For this review, take the finished solid that the model builds, in its own axes (mm). Face numbers are marked on the shaded views. A direction names the side the tool comes from. Round coordinates to 2 decimals unless told otherwise and drop trailing zeros. Order: outer loops, then holes, each group sorted by start corner. A loop starts at its lowest first (then second) coordinate and runs counter-clockwise, first axis right, second up. Notation, with made-up numbers: M 8.5,-12 L 43.5,-12 A10 cw 43.5,-2 Z; hole C -35.5,3.5 d10. An arc over 180 degrees is marked long. Put each result on its own line as item: value.
from build123d import *

# Parameters (mm, degrees)
F1_DEPTH       = 101.6
F3_D           = 9.525
F3_DEPTH       = 15.875
F3_CBORE_D     = 9.525
F3_CBORE_DEPTH = 9.525
F3_TIP         = 2.8615986981
F5_D           = 9.525
F5_CBORE_D     = 12.7
F5_CBORE_DEPTH = 12.7
F6_W           = 38.1
F6_H           = 38.1
F7_DEPTH       = 57.913
F8_R           = 9.525
F9_DEPTH       = 31.751


with BuildPart() as f1:
    # F0 (on Right) → F1 (new body)
    with BuildSketch(Plane.YZ):
        with BuildLine():
            Line((-18.288, 0), (-32.512, 0))
            Line((-32.512, 0), (-32.512, -31.75))
            Line((-32.512, -31.75), (-26.162, -31.75))
            ThreePointArc((-26.162, -31.75), (-24.3021280605, -27.2598719395), (-19.812, -25.4))
            Line((-19.812, -25.4), (19.812, -25.4))
            ThreePointArc((19.812, -25.4), (24.3021280605, -27.2598719395), (26.162, -31.75))
            Line((26.162, -31.75), (32.512, -31.75))
            Line((32.512, -31.75), (32.512, 0))
            Line((32.512, 0), (18.288, 0))
            Line((18.288, 0), (18.288, 6.35))
            Line((18.288, 6.35), (25.4, 6.35))
            Line((25.4, 6.35), (25.4, 38.1))
            Line((25.4, 38.1), (19.05, 38.1))
            Line((19.05, 38.1), (3.302, 22.352))
            Line((3.302, 22.352), (3.302, 16.002))
            Line((3.302, 16.002), (-3.302, 16.002))
            Line((-3.302, 16.002), (-3.302, 22.352))
            Line((-3.302, 22.352), (-19.05, 38.1))
            Line((-19.05, 38.1), (-25.4, 38.1))
            Line((-25.4, 38.1), (-25.4, 6.35))
            Line((-25.4, 6.35), (-18.288, 6.35))
            Line((-18.288, 6.35), (-18.288, 0))
        make_face()
    extrude(amount=-F1_DEPTH)

    # F3
    with Locations(Plane.YZ):
        with Locations((0, -9.525)):
            CounterBoreHole(F3_D / 2, F3_CBORE_D / 2, F3_CBORE_DEPTH, depth=F3_DEPTH)
            with Locations((0, 0, -(F3_DEPTH + F3_TIP / 2))):  # 118° drill point
                Cone(0, F3_D / 2, F3_TIP, mode=Mode.SUBTRACT)

    # F5 (through all)
    with Locations(Plane.XZ.offset(32.512)):
        with Locations((-50.8, -15.875)):
            CounterBoreHole(F5_D / 2, F5_CBORE_D / 2, F5_CBORE_DEPTH)

    # F6 (on face) → F7 (cut, through all)
    with BuildSketch(Plane.XZ.offset(25.4)):
        with Locations((-50.8, 19.05)):
            Rectangle(F6_W, F6_H)
    extrude(amount=-F7_DEPTH, mode=Mode.SUBTRACT)

    # F8 (on face) → F9 (cut, through all)
    with BuildSketch(Plane.XY):
        with Locations((-50.8, 0)):
            Circle(F8_R)
    extrude(amount=-F9_DEPTH, mode=Mode.SUBTRACT)


solid = f1.part
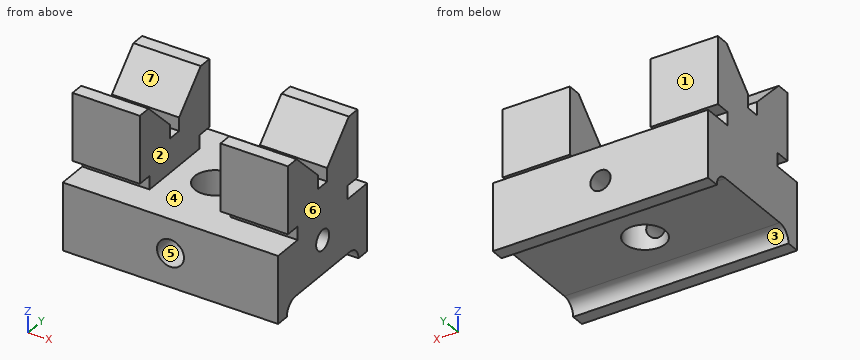
(1) Add section A-A on z = 4. Give the boundary of the cut face in (x, y).
A:
outline: M -101.6,-18.29 L -69.85,-18.29 L -69.85,18.29 L -101.6,18.29 Z; M -31.75,-18.29 L 0,-18.29 L 0,18.29 L -31.75,18.29 Z
(2) Add section B-B on z = 33. Give the boundary of the cut face in (x, y).
A:
outline: M -101.6,-25.4 L -69.85,-25.4 L -69.85,-13.95 L -101.6,-13.95 Z; M -101.6,13.95 L -69.85,13.95 L -69.85,25.4 L -101.6,25.4 Z; M -31.75,-25.4 L 0,-25.4 L 0,-13.95 L -31.75,-13.95 Z; M -31.75,13.95 L 0,13.95 L 0,25.4 L -31.75,25.4 Z
(3) To check wall thickness, follow L1, parallel to Z at x = -10.75, y = 0; L2, parallel to X at y = -6, z = 5; L3, parallel to Z at x = -92, y = 1. State the ranges of each line that lie inside material, in increasing order.
A:
L1: z = -25.4 to -14.29, -4.76 to 16
L2: x = -101.6 to -69.85, -31.75 to 0
L3: z = -25.4 to 16
(4) Add section D-D on y = -7. Give the boundary of the cut face in (x, z), then the cut area to 3 significant figures.
A:
outline: M -101.6,-25.4 L -57.26,-25.4 L -57.26,0 L -69.85,0 L -69.85,26.05 L -101.6,26.05 Z; M -44.34,-25.4 L 0,-25.4 L 0,26.05 L -31.75,26.05 L -31.75,0 L -44.34,0 Z
area: 3,910 mm2
(5) Draft analysis for pull direction Z (two halves, no side actions). For the marked faces 4, 5, 6 and 7, state which applies: released by +Z, released by -Z, zero draft, split by the parting line, or undercut.
A:
face 4: undercut
face 5: undercut
face 6: zero draft
face 7: released by +Z
(6) Add section C-C on x = -50.8. State how many separate pieces and enclosed holes the cut face has, then the cut area to 3 significant figures.
A:
separate pieces: 4
enclosed holes: 0
area: 787 mm2
(7) For the marked faces 1, 2 and 3, list the 3-axis set-ups (+Z, -Z, +X, -X, +Y, -Y) from which the entire face can be reached by the end or side of a thin tool; tool diameter is ignored.
A:
face 1: +Z, +X, -X, +Y
face 2: +Z, +Y, -Y
face 3: -Z, +X, -X
(8) Insertion check: pin 1 Ø5 at (x, z) = (-11.5, 3.5) entering from -Y; pin 2 Ø12 at (x, z) = (-30, 22.5) entering from -Y; pin 3 Ø1 at (x, y) = (-68.5, 24) entering from +Z. Each pin has a flat end and moves straight along its axis. Give the tip position at first contact, or say it passes through.
A:
pin 1: stops at y = -18.29
pin 2: stops at y = -25.4
pin 3: stops at z = 0
